Work out the finished part from the listing and answer in its coordinate system (mm). A direction names the side the tool comes from. Give positions to 0.01 mm unless a question says otherwise; leave off trailing zeros. Write each loop counter-clockwise with the first axis right and the second up, starting at its lowest first coordinate (ties: lowest second). Pieces come first, ordered by that corner, then holes.
1) Find section A-A (x = 0). Determine the outline of the cut face in (y, z).
2) Find section C-C (y = -0.55). Determine the outline of the cut face in (x, z), plus the area to 3 significant figures.
3) Find section B-B (z = 6). Determine the outline of the cut face in (x, y).
4) Determine the mould class of faces 3 (the face through (-11.99, -2.46, 0.53)), 4 (the face through (0, -5, 0)), 5 (the face through (9.2, -1.48, 0.05)) for opening direction Z: pulls with the +Z half, pulls with the -Z half, needs draft (parallel to the pull), parting line crosses it, or undercut.
5) Straight lines are drawn through the part: probe 1 along Z at (x, y) = (0, -1.5); probe 2 along X at (y, z) = (-3.75, -1); probe 3 along Z at (x, y) = (0, -3.75). For each, find the intervals that lie inside material, in ascending order.
6) Given pin 1 Ø2 at (x, z) = (8, 0) entering from -Y; pin 2 Ø1 at (x, y) = (2.5, -2) entering from +Z; pin 3 Ø3 at (x, z) = (0, 6) entering from -Y, each flat-ended and moving along its own axis, determine where each tip first touches the part or whether it passes through.
7) A tool of negligible diameter and unlimited length cuts with its end or side. For faces 1 (the face through (0, 0, 0)), 2 (the face through (-10.5, -4, 0.1)), from which of +Z, -Z, +X, -X, +Y, -Y can it reach the whole face along a straight path? Write none if from no direction.
8) Find section D-D (y = -3.8). Determine the outline of the cut face in (x, z).
```python
from build123d import *

# Parameters (mm, degrees)
F0_R     = 12
F1_DEPTH = 5
F2_R     = 1.2
F3_DEPTH = 5
F4_R     = 2.5
F5_DEPTH = 2


with BuildPart() as f1:
    # F0 (on Front) → F1 (new body)
    with BuildSketch(Plane.XZ):
        Circle(F0_R)
    extrude(amount=F1_DEPTH)

    # F2 (on face) → F3 (cut)
    with BuildSketch(Plane(origin=(0, 0, 0), x_dir=(-1, 0, 0), z_dir=(0, 1, 0))):
        with Locations((8, 0)):
            Circle(F2_R)
        with Locations((-8, 0)):
            Circle(F2_R)
        with Locations((0, 6)):
            Circle(F2_R)
    extrude(amount=-F3_DEPTH, mode=Mode.SUBTRACT)

    # F4 (on face) → F5 (cut)
    with BuildSketch(Plane.XZ.offset(5)):
        with Locations((0, 6)):
            Circle(F4_R)
        with Locations((8, 0)):
            Circle(F4_R)
        with Locations((-8, 0)):
            Circle(F4_R)
    extrude(amount=-F5_DEPTH, mode=Mode.SUBTRACT)


solid = f1.part
```
Results:
1. outline: (-5, -12) - (0, -12) - (0, 4.8) - (-3, 4.8) - (-3, 3.5) - (-5, 3.5) - close; (-5, 8.5) - (-3, 8.5) - (-3, 7.2) - (0, 7.2) - (0, 12) - (-5, 12) - close
2. outline: circle Ø24 at (0, 0); hole circle Ø2.4 at (-8, 0); hole circle Ø2.4 at (0, 6); hole circle Ø2.4 at (8, 0)
2. area: 439 mm2
3. outline: (-10.39, -5) - (-2.5, -5) - (-2.5, -3) - (-1.2, -3) - (-1.2, 0) - (-10.39, 0) - close; (1.2, -3) - (2.5, -3) - (2.5, -5) - (10.39, -5) - (10.39, 0) - (1.2, 0) - close
4. face 3: parting line crosses it
4. face 4: needs draft
4. face 5: undercut
5. probe 1: z = -12 to 4.8, 7.2 to 12
5. probe 2: x = -11.96 to -10.29, -5.71 to 5.71, 10.29 to 11.96
5. probe 3: z = -12 to 3.5, 8.5 to 12
6. pin 1: passes through
6. pin 2: stops at z = 11.83
6. pin 3: stops at y = -3
7. face 1: +Z, -Z, +X, -X, +Y
7. face 2: -Y
8. outline: circle Ø24 at (0, 0); hole circle Ø5 at (-8, 0); hole circle Ø5 at (0, 6); hole circle Ø5 at (8, 0)
